Verification items for the finished model (mm, model axes). Face numbers are marked on the shaded views. Give positions to 0.01 mm unless a question says otherwise; leave off trailing zeros. Write each loop counter-clockwise with the first axis right and the second up, starting at its lowest first coordinate (ties: lowest second). Pieces come first, ordered by that corner, then holes. Notation, with made-up numbers: (-30, 83.5) - (24, 83.5) arc R26 ccw to (24, 106.5) - close; hole circle Ø8 at (89, 77). An arc over 180 degrees is marked (long way). Answer as a JSON object with one key per item and string values. Group by question number.
Item 1: Draft check along X on the marked faces 1, 2 and 3. Enter one of: +X half, -X half, draft (parallel to the pull), parting line (faces both ways), or undercut.
Item 2: Sectioned sample at A-A, the plane y = 0. Record the boundary of the cut face in (x, z).
Item 3: Go/stop test with flat-tipped pins: pin 1 (5 mm diameter, centred on y = 7, z = 10.5, fed in from +X); pin 2 (1.5 mm diameter, centred on y = -12, z = 3, fed in from -X); pin 3 (5 mm diameter, centred on y = 11, z = 8.5, fed in from -X); pin 4 (4 mm diameter, centred on x = -2.5, y = 8, fed in from -Z). Record where each tip stops, or that it passes through.
Item 4: Sectioned sample at C-C, the plane z = 8.5. Record the boundary of the cut face in (x, y).
Item 5: Scan lines: line 1 along X through (y, z) = (0, 10.25); line 2 along Z through (x, y) = (10, -12); line 3 along Y through (x, z) = (-3, 11). Record each from-to range of solid material in increasing order. Write a range as [from, to].
```python
from build123d import *

# Parameters (mm, degrees)
ESQUISSE1_W     = 1.75
ESQUISSE1_H     = 2
ESQUISSE1_W_2   = 15
ESQUISSE1_H_2   = 7
CHANFREIN1_SIZE = 0.75


with BuildPart() as part:
    # Esquisse1 → Révolution1 (revolve)
    with BuildSketch(Plane(origin=(0, 0, 0), x_dir=(0, 0, -1), z_dir=(1, 0, 0))):
        Polygon((-15, 15), (-15, 11), (0, 11), (0, 15), (-1.75, 15), (-13.25, 15), align=None)
        with Locations((-14.125, 16)):
            Rectangle(ESQUISSE1_W, ESQUISSE1_H)
        with Locations((-0.875, 16)):
            Rectangle(ESQUISSE1_W, ESQUISSE1_H)
        with Locations((-7.5, 7.5)):
            Rectangle(ESQUISSE1_W_2, ESQUISSE1_H_2)
    revolve(axis=Axis((0, 0, 15), (0, 0, -1)))

    # Chanfrein1
    chanfrein1_edges = [part.edges().sort_by_distance(p)[0] for p in [
        (0, -17, 1.75),
        (0, -17, 13.25),
    ]]
    chamfer(chanfrein1_edges, length=CHANFREIN1_SIZE)


solid = part.part
```
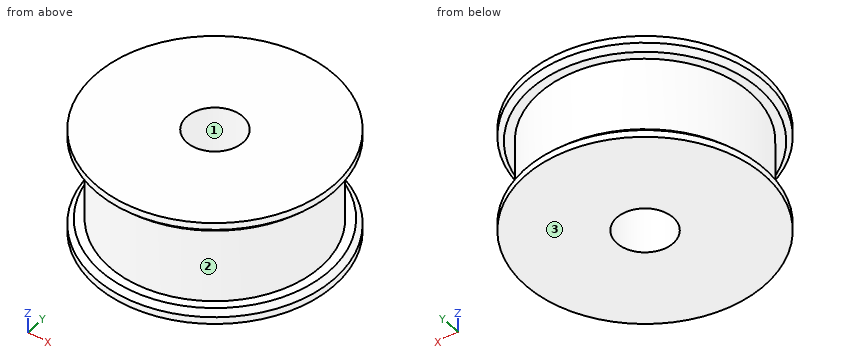
Geometry check:
{
 "1": {"face 1": "undercut", "face 2": "parting line", "face 3": "draft"},
 "2": {"outline": "(-17, 0) - (-4, 0) - (-4, 15) - (-17, 15) - (-17, 14) - (-16.25, 13.25) - (-15, 13.25) - (-15, 1.75) - (-16.25, 1.75) - (-17, 1) - close; (4, 0) - (17, 0) - (17, 1) - (16.25, 1.75) - (15, 1.75) - (15, 13.25) - (16.25, 13.25) - (17, 14) - (17, 15) - (4, 15) - close"},
 "3": {"pin 1": "x = 14.31", "pin 2": "x = -9.92", "pin 3": "x = -12.36", "pin 4": "z = 0"},
 "4": {"outline": "circle Ø30 at (0, 0); hole circle Ø8 at (0, 0)"},
 "5": {"line 1": "[-15, -4], [4, 15]", "line 2": "[0, 1.75], [13.25, 15]", "line 3": "[-14.7, -2.65], [2.65, 14.7]"}
}
